Source: CAD feature listing. Evaluate the final solid. Frame: model axes, mm. A direction names the side the tool comes from. Give positions to 0.01 mm unless a question says otherwise; leave off trailing zeros. Write each loop counter-clockwise with the first axis right and the second up, starting at its lowest first coordinate (ties: lowest second). Pieces come first, ordered by that corner, then holes. Notation, with made-up numbers: M -21,75.25 L 7,75.25 A18 ccw 7,90.25 Z; hole C -34.75,-34.5 d9. An arc over 180 degrees is marked long. Return JSON: item names as keys, results as strings.
```python
from build123d import *

# Parameters (mm, degrees)
F1_DEPTH       = 8
F3_D           = 4.4
F3_CSINK_D     = 8.96
F3_CSINK_ANGLE = 90


with BuildPart() as f1:
    # F0 (on Top) → F1 (new body)
    with BuildSketch(Plane.XY):
        with BuildLine():
            Line((-10, 0), (-5, 0))
            ThreePointArc((-5, 0), (-1.4644660941, -1.4644660941), (0, -5))
            Line((0, -5), (0, -10))
            Line((0, -10), (8, -10))
            Line((8, -10), (8, 3))
            Line((8, 3), (-10, 3))
            Line((-10, 3), (-10, 0))
        make_face()
    extrude(amount=F1_DEPTH)

    # F3 (through all)
    with Locations(Plane(origin=(0, 3, 0), x_dir=(-1, 0, 0), z_dir=(0, 1, 0))):
        with Locations((-4, 4)):
            CounterSinkHole(F3_D / 2, F3_CSINK_D / 2, counter_sink_angle=F3_CSINK_ANGLE)


solid = f1.part
```
1) Set-up query: faces 4 (the face through (6, -10, 6)), 5 (the face through (0, -7, 4)). Return all of +Z, -Z, +X, -X, +Y, -Y with unobstructed straight access to the full face (end or side cutting, diameter ignored); none if empty.
Numbers:
{"face 4": "+Z, -Z, +X, -X, -Y", "face 5": "+Z, -Z, -X, -Y"}
2) Cut plane D-D, the plane x = -8. Return the cut outline in (y, z), then the cut area to 3 significant figures.
Numbers:
{"outline": "M 0,0 L 3,0 L 3,8 L 0,8 Z", "area": "24.0 mm²"}
3) Draft query along X for faces 1 (the face through (-10, 2, 4)), 2 (the face through (6.032, -4.715, 3.157)), 3 (the face through (1, -2, 8)). Return one class per face: released by +X, released by -X, zero draft, split by the parting line, or undercut.
Numbers:
{"face 1": "released by -X", "face 2": "undercut", "face 3": "zero draft"}
4) Contact query for flat-ended pins moving along their axis: pin 1 Ø2 at (y, z) = (-7.5, 3) entering from -X; pin 2 Ø1.5 at (x, z) = (-7.5, 5) entering from -Y; pin 3 Ø2 at (x, z) = (-3, 1.5) entering from -Y. Output: stop coordinate, or through.
Numbers:
{"pin 1": "stops at x = 0", "pin 2": "stops at y = 0", "pin 3": "stops at y = -1"}
5) Line query: line 1 (Z direction, x = 4, y = -4.75); line 2 (Y direction, x = -7.25, z = 1); line 3 (X direction, y = -8.75, z = 4.75). Output: solid intervals per line, ascending. Write a range as [from, to].
Numbers:
{"line 1": "z = [0, 1.8], [6.2, 8]", "line 2": "y = [0, 3]", "line 3": "x = [0, 1.93], [6.07, 8]"}
6) Cut plane C-C, the plane z = 4. Return the cut outline in (x, y).
Numbers:
{"outline": "M -10,0 L -5,0 A5 cw 0,-5 L 0,-10 L 1.8,-10 L 1.8,0.72 L -0.48,3 L -10,3 Z; M 6.2,-10 L 8,-10 L 8,2.52 L 6.2,0.72 Z"}
7) Cut plane B-B, the plane y = 2. Return the cut outline in (x, z), then the cut area to 3 significant figures.
Numbers:
{"outline": "M -10,0 L 8,0 L 8,8 L -10,8 Z; hole C 4,4 d6.96", "area": "106 mm²"}
8) Cut plane A-A, the plane x = 4. Return the cut outline in (y, z).
Numbers:
{"outline": "M -10,0 L 2.52,0 L 0.72,1.8 L -10,1.8 Z; M -10,6.2 L 0.72,6.2 L 2.52,8 L -10,8 Z"}
